The listing builds one solid part. Answer for the finished solid, in the listing's coordinates (mm). A direction names the side the tool comes from. Give positions to 0.01 mm unless a question says otherwise; leave off trailing zeros. Loops run counter-clockwise (first coordinate to the right, second up) from the corner with the lowest first, then second, coordinate; pieces in that order, holes last. Notation, with made-up numbers: (81.5, 46) - (89.5, 46) arc R16 ccw to (89.5, 67) - close; hole circle Ø11 at (61, -17.5). An arc over 180 degrees is marked (long way). One line per item, written item: value. Start each with the question number.
Solid Edge part; units mm, degrees
sketch "Sketch1" plane through (0, 0, 0) normal (1, 0, 0) x (0, 1, 0)
  line L0 (37.2104, 138.8713) -> (37.2104, 188.8713)
  spline S0 degree 3 poles (100, 180) (97.8773, 199.692) (72.5701, 247.7114) (42.0437, 203.6951) (37.2104, 188.8713) knots 0 0 0 0 0.527303 1 1 1 1
  line L1 (100, 0) -> (100, 180)
  line L2 (0, 0) -> (100, 0)
  line L3 (0, 0) -> (37.2104, 138.8713)
extrude "Protrusion1" add sketch "Sketch1" against normal blind 10
mirror "Mirror1" about plane through (-640, 0, 0) normal (1, 0, 0) of "Protrusion1"
sketch "Sketch2" plane through (-10, 50, 112.439) normal (-1, 0, 0) x (0, -1, 0)
  line L0 (-50, -112.439) -> (-50, 67.561)
  spline S0 degree 3 poles (-50, 67.561) (-47.8885, 87.149) (-34.6735, 112.3063) (-19.9715, 112.3063) knots 0 0 0 0 1 1 1 1
  line L1 (-19.9715, 112.3063) -> (-19.975, 102.3046)
  spline S1 degree 3 poles (-40, 66.9953) (-39.5373, 70.9153) (-38.5008, 75.3255) (-35.4559, 84.1103) (-33.4066, 88.4861) (-29.9959, 93.9577) (-28.8084, 95.6011) (-26.4539, 98.375) (-25.2871, 99.5054) (-23.1744, 101.1643) (-22.2404, 101.6859) (-21.1658, 102.1077) (-20.8601, 102.1932) (-20.3629, 102.2886) (-20.1637, 102.3046) (-19.975, 102.3046) knots 0 0 0 0 0.243507 0.243507 0.497563 0.497563 0.62459 0.62459 0.751618 0.751618 0.878646 0.878646 0.94216 0.94216 1 1 1 1
  line L2 (-40, -102.439) -> (-40, 66.9953)
  line L3 (36.9677, -102.439) -> (-40, -102.439)
  line L4 (50, -112.439) -> (36.9677, -102.439)
  line L5 (50, -112.439) -> (-50, -112.439)
extrude "Protrusion3" add sketch "Sketch2" along normal up to next
fillet "Round_1" radius 50 1 edges at (-640, 90, 10)
fillet "Round_2" radius 50 1 edges at (-640, 100, 0)
sketch "Sketch3" plane through (-540, 100, 115) normal (0, 1, 0) x (-1, 0, 0)
  line L0 (-50, 48.6858) -> (-40, 48.6858)
  line L1 (-40, 48.6858) -> (-40, -51.3142)
  line L2 (-40, -51.3142) -> (-50, -51.3142)
  line L3 (-50, -51.3142) -> (-50, 48.6858)
  line L4 (250, 48.6858) -> (240, 48.6858)
  line L5 (240, 48.6858) -> (240, -51.3142)
  line L6 (240, -51.3142) -> (250, -51.3142)
  line L7 (250, -51.3142) -> (250, 48.6858)
  dimension "D1" = 50
extrude "Protrusion4" add sketch "Sketch3" along normal blind 150
extrude "Cutout1" [suppressed]
sketch "Sketch4" plane through (-490, 175, 113.6858) normal (1, 0, 0) x (0, 1, 0)
  circle A0 centre (25, 0) radius 30
  dimension "D1" = 25
extrude "ExtrudedProtrusion_5" add sketch "Sketch4" along normal blind 50
mirror "Mirror2" about plane through (-640, 175, 113.6858) normal (-1, 0, 0) of "ExtrudedProtrusion_5"
1. Flat-ended cylindrical pins translate along their axes: pin 1 (2 mm diameter, centred on x = -614.5, z = 104.5, fed in from -Y); pin 2 (5 mm diameter, centred on x = -1275.5, z = 102.5, fed in from +Y); pin 3 (8 mm diameter, centred on x = -494, y = 140, fed in from +Z). Find the tip coordinate at first contact, or state that the pin passes through.
2. For faces 1 (the flat face through (-631, 26, 10)), 2 (the flat face through (-490, 157, 113)), 3 (the cylindrical face through (-648.82, 75.742, 25.036)), 4 (the flat face through (-780, 174, 114)), 5 (the flat face through (-790, 157, 113)), determine the directions among +Z, -Z, +X, -X, +Y, -Y from which every point of the face is accessible in a straight line to the end or side of a thin tool.
3. Determine the mould class of faces 6 (the flat face through (-1270, 54, 111)), 7 (the flat face through (-1275.07, 18.866, 70.408)), 8 (the flat face through (-1280, 60, 95)) for opening direction X: released by +X, released by -X, zero draft, split by the parting line, or undercut.
4. A cutting plane is placed at A-A (y = 200). Determine the outline of the cut face in (x, z), plus the area to 3 significant figures.
5. A cutting plane is placed at B-B (z = 101.5). Determine the outline of the cut face in (x, y).
6. Find the intervals of material crossed by L1, parallel to X at y = 61, z = 41.5; L2, parallel to X at y = 198, z = 121; L3, parallel to Y at x = -810, z = 149, in increasing order. Write a range as [from, to].
Results below:
1. pin 1: stops at y = 90
1. pin 2: stops at y = 100
1. pin 3: stops at z = 163.69
2. face 1: +Z, -Y
2. face 2: +X
2. face 3: -Y
2. face 4: +Z, -Z, +Y
2. face 5: -X
3. face 6: undercut
3. face 7: zero draft
3. face 8: released by -X
4. outline: (-840, 83.69) - (-790, 83.69) - (-790, 63.69) - (-780, 63.69) - (-780, 163.69) - (-790, 163.69) - (-790, 143.69) - (-840, 143.69) - close; (-500, 63.69) - (-490, 63.69) - (-490, 83.69) - (-440, 83.69) - (-440, 143.69) - (-490, 143.69) - (-490, 163.69) - (-500, 163.69) - close
4. area: 8,000 mm^2
5. outline: (-1280, 27.2) - (-1270, 27.2) - (-1270, 90) - (-10, 90) - (-10, 27.2) - (0, 27.2) - (0, 100) - (-490, 100) - (-490, 172.59) - (-440, 172.59) - (-440, 227.41) - (-490, 227.41) - (-490, 250) - (-500, 250) - (-500, 100) - (-780, 100) - (-780, 250) - (-790, 250) - (-790, 227.41) - (-840, 227.41) - (-840, 172.59) - (-790, 172.59) - (-790, 100) - (-1280, 100) - close
6. L1: x = [-1280, -1270], [-10, 0]
6. L2: x = [-840, -780], [-500, -440]
6. L3: y = [90, 100]
